Part model, mm, in its own coordinate system. A direction names the side the tool comes from. Round coordinates to 2 decimals unless told otherwise and drop trailing zeros. Order: outer loops, then holes, each group sorted by start corner. A loop starts at its lowest first (then second) coordinate and runs counter-clockwise, first axis right, second up. Notation, with made-up numbers: (79.25, -7.5) - (124.25, -7.5) arc R19 ccw to (124.25, -0.5) - close; hole circle Ø5 at (-19.5, 19). An arc over 180 degrees is marked (long way). Answer as a JSON object with one key per item and string values.
```python
from build123d import *

# Parameters (mm, degrees)
SKETCH2_R           = 2.5
SKETCH2_R_2         = 3
SKETCH2_R_3         = 2
BOSS_EXTRUDE1_DEPTH = 6


with BuildPart() as part:
    # Sketch2 → Boss-Extrude1 (new body)
    with BuildSketch(Plane(origin=(0, 1180.436182905, 0), x_dir=(1, 0, 0), z_dir=(0, 1, 0))):
        Polygon((791.275007127, -1801.911067916), (791.275007127, -1920.911067916), (772.275007127, -1920.911067916), (772.275007127, -1972.911067916), (850.275007127, -1972.911067916), (850.275007127, -1920.911041247), (831.275007127, -1920.911049835), (831.340606325, -1801.911067916), align=None)
        with Locations(Location((811.275007127, -1946.911067916, 0), (0, 0, 270))):
            Circle(SKETCH2_R, mode=Mode.SUBTRACT)
        with Locations(Location((784.275007127, -1930.911067916, 0), (0, 0, 270))):
            Circle(SKETCH2_R_2, mode=Mode.SUBTRACT)
        with Locations(Location((784.275007127, -1962.911067916, 0), (0, 0, 270))):
            Circle(SKETCH2_R_2, mode=Mode.SUBTRACT)
        with Locations(Location((838.275007127, -1930.911067916, 0), (0, 0, 270))):
            Circle(SKETCH2_R_2, mode=Mode.SUBTRACT)
        with Locations(Location((838.275007127, -1962.911067916, 0), (0, 0, 270))):
            Circle(SKETCH2_R_2, mode=Mode.SUBTRACT)
        with Locations(Location((800.275007127, -1921.911067916, 0), (0, 0, 270))):
            Circle(SKETCH2_R_3, mode=Mode.SUBTRACT)
        with Locations(Location((800.275007127, -1821.911067916, 0), (0, 0, 270))):
            Circle(SKETCH2_R_3, mode=Mode.SUBTRACT)
        with Locations(Location((822.275007127, -1921.911067916, 0), (0, 0, 270))):
            Circle(SKETCH2_R_3, mode=Mode.SUBTRACT)
        with Locations(Location((822.275007127, -1821.911067916, 0), (0, 0, 270))):
            Circle(SKETCH2_R_3, mode=Mode.SUBTRACT)
    extrude(amount=BOSS_EXTRUDE1_DEPTH)


solid = part.part
```
Item 1: Cut at B-B (x = 777.5). Write the cut outline in (y, z), plus the area to 3 significant figures.
Taken from the geometry:
{"outline": "(1180.44, 1920.91) - (1186.44, 1920.91) - (1186.44, 1972.91) - (1180.44, 1972.91) - close", "area": "312 mm2"}
Item 2: Tool access for faces 4 (the flat face through (782, 1183, 1920.911)), 5 (the flat face through (772.275, 1183, 1947)): list every direction of +Z, -Z, +X, -X, +Y, -Y with a clear straight run to the whole face (end or side of a thin tool).
Taken from the geometry:
{"face 4": "-Z, -X, +Y, -Y", "face 5": "+Z, -Z, -X, +Y, -Y"}
Item 3: Cut at C-C (z = 1839.5). Write the cut outline in (x, y) (3 decimals).
Taken from the geometry:
{"outline": "(791.275, 1180.436) - (831.32, 1180.436) - (831.32, 1186.436) - (791.275, 1186.436) - close"}
Item 4: Cut at A-A (y = 1182.65). State how many separate pieces and enclosed holes the cut face has, plus the area to 3 significant figures.
Taken from the geometry:
{"separate pieces": "1", "enclosed holes": "9", "area": "8,640 mm2"}
Item 5: Two-plate mould, pull along X, no slides. Class faces 1 (the flat face through (841, 1183, 1920.911)), 2 (the cylindrical face through (800.876, 1183.394, 1823.819)), 3 (the flat face through (850.275, 1183, 1947)): pulls with the +X half, pulls with the -X half, needs draft (parallel to the pull), parting line crosses it, or undercut.
Taken from the geometry:
{"face 1": "needs draft", "face 2": "undercut", "face 3": "pulls with the +X half"}
Item 6: Drop flat-ended pins along their axis: P1, Ø1.8, axis at y = 1183, z = 1840.5, coming from the -X side (3 decimals); P2, Ø5.5, axis at x = 784.28, z = 1930.91, coming from the +Y side; P3, Ø1.8, axis at x = 837, y = 1184, coming from the -Z side; P4, Ø1, axis at y = 1185, z = 1842, coming from the +X side. Give the stop position or say it passes through.
Taken from the geometry:
{"P1": "x = 791.275", "P2": "through", "P3": "z = 1920.91", "P4": "x = 831.32"}
Item 7: Probe L1, parallel to Z at x = 824, y = 1181.3; L2, parallel to Z at x = 811, y = 1181.7; L3, parallel to Z at x = 840, y = 1181.65. List the from-to ranges inside material, lowest first. Write a range as from..to.
Taken from the geometry:
{"L1": "1801.91..1820.9, 1822.92..1920.9, 1922.92..1972.91", "L2": "1801.91..1944.43, 1949.4..1972.91", "L3": "1920.91..1928.46, 1933.37..1960.46, 1965.37..1972.91"}
